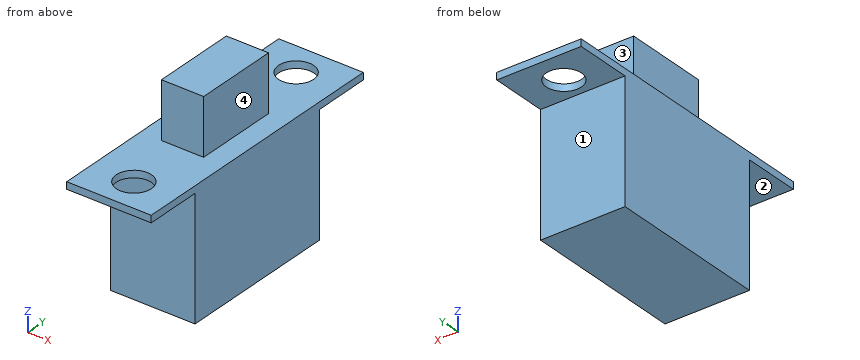
from build123d import *

# Parameters (mm, degrees)
SKETCH1_W           = 6
SKETCH1_H           = 19.6
BOSS_EXTRUDE1_DEPTH = 0.5
SKETCH2_R           = 1.25
CUT_EXTRUDE1_DEPTH  = 1
SKETCH3_W           = 6
SKETCH3_H           = 11.5
BOSS_EXTRUDE2_DEPTH = 9.1
SKETCH6_W           = 3
SKETCH6_H           = 6
BOSS_EXTRUDE3_DEPTH = 4


with BuildPart() as part:
    # Sketch1 → Boss-Extrude1 (new body)
    with BuildSketch(Plane.XY):
        with Locations((21.125833333, 0.952916667)):
            Rectangle(SKETCH1_W, SKETCH1_H)
    extrude(amount=BOSS_EXTRUDE1_DEPTH)

    # Sketch2 → Cut-Extrude1 (cut)
    with BuildSketch(Plane(origin=(0, 0, 0), x_dir=(-1, 0, 0), z_dir=(0, 0, -1))):
        with Locations((-21.125833333, 8.452916667)):
            Circle(SKETCH2_R)
        with Locations((-21.125833333, -6.547083333)):
            Circle(SKETCH2_R)
    extrude(amount=-CUT_EXTRUDE1_DEPTH, mode=Mode.SUBTRACT)



with BuildPart() as body_2:
    # Sketch3 → Boss-Extrude2 (new body)
    with BuildSketch(Plane.XY.offset(0.5)):
        with Locations((21.125833333, 0.952916667)):
            Rectangle(SKETCH3_W, SKETCH3_H)
    extrude(amount=-BOSS_EXTRUDE2_DEPTH)


with BuildPart() as part_1:
    add(part.part)

    add(body_2.part)  # Boss-Extrude3 merges body 2
    # Sketch6 → Boss-Extrude3 (add)
    with BuildSketch(Plane.XY.offset(0.5)):
        with Locations((21.125833333, 0.952916667)):
            Rectangle(SKETCH6_W, SKETCH6_H)
    extrude(amount=BOSS_EXTRUDE3_DEPTH)


solid = part_1.part
Input: part model. Units: mm. Frame: model coordinates. Face numbers are marked on the shaded views. A direction names the side the tool comes from. Coordinates: 2 decimals unless noted, no trailing zeros. Loops run counter-clockwise (first coordinate to the right, second up) from the corner with the lowest first, then second, coordinate; pieces in that order, holes last.
(1) Section D-D on x = 20.3. Return the cut outline in (y, z), then the cut area to 3 significant figures.
(2) Set-up query: the marked faces 1, 2, 3 and 4. Return all of +Z, -Z, +X, -X, +Y, -Y with unobstructed straight access to the full face (end or side cutting, diameter ignored); none if empty.
(3) Section B-B on x = 23.55. Return the cut outline in (y, z), then the cut area to 3 significant figures.
(4) Section C-C on y = -5.75. Return the cut outline in (x, z).
(5) First-contact query: pin 1 Ø1.8 at (x, z) = (21.5, -6) entering from +Y; pin 2 Ø1.5 at (y, z) = (2, 1.5) entering from +X; pin 3 Ø3 at (x, y) = (21.5, 9) entering from -Z. Flat tips, straight axial feed; report the tip coordinate or a pass-through.
(6) Section A-A on y = 2.75. Return the cut outline in (x, z), then the cut area to 3 significant figures.
(7) Material intervals for probe 1 along Y at (x, z) = (21.65, 3.5); probe 2 along Z at (x, y) = (18.65, 7); probe 3 along Z at (x, y) = (19.75, 6.5), sorted ascending.
Data:
1. outline: (-8.85, 0) - (-7.49, 0) - (-7.49, 0.5) - (-8.85, 0.5) - close; (-5.61, 0) - (-4.8, 0) - (-4.8, -8.6) - (6.7, -8.6) - (6.7, 0) - (7.51, 0) - (7.51, 0.5) - (3.95, 0.5) - (3.95, 4.5) - (-2.05, 4.5) - (-2.05, 0.5) - (-5.61, 0.5) - close; (9.39, 0) - (10.75, 0) - (10.75, 0.5) - (9.39, 0.5) - close
1. area: 131 mm2
2. face 1: -Z, +X, -X, +Y
2. face 2: -Z, +X, -X, -Y
2. face 3: +Z, +X, -X, +Y
2. face 4: +Z, +X, +Y, -Y
3. outline: (-8.85, 0) - (-4.8, 0) - (-4.8, -8.6) - (6.7, -8.6) - (6.7, 0) - (10.75, 0) - (10.75, 0.5) - (-8.85, 0.5) - close
3. area: 109 mm2
4. outline: (18.13, 0) - (20.16, 0) - (20.16, 0.5) - (18.13, 0.5) - close; (22.09, 0) - (24.13, 0) - (24.13, 0.5) - (22.09, 0.5) - close
5. pin 1: stops at y = 6.7
5. pin 2: stops at x = 22.63
5. pin 3: stops at z = 0
6. outline: (18.13, -8.6) - (24.13, -8.6) - (24.13, 0.5) - (22.63, 0.5) - (22.63, 4.5) - (19.63, 4.5) - (19.63, 0.5) - (18.13, 0.5) - close
6. area: 66.6 mm2
7. probe 1: y = -2.05 to 3.95
7. probe 2: z = 0 to 0.5
7. probe 3: z = -8.6 to 0.5
